Check sheet for the modelled part. Datum: model origin and axes. Units: mm. Coordinates: 2 decimals unless noted, no trailing zeros. Loops run counter-clockwise (first coordinate to the right, second up) from the corner with the lowest first, then second, coordinate; pieces in that order, holes last. Notation, with made-up numbers: M 77,77.25 L 81,77.25 A21 cw 81,105.25 Z; hole C -18.5,81 d6. An arc over 180 degrees is marked long. Use CSV: the item, a comma, the result in double quotes. Start each with the question number.
(1) Go/stop test with flat-tipped pins: pin 1 Ø1.4 at (x, z) = (38.5, 3.5) entering from +Y; pin 2 Ø4 at (x, z) = (37, 3.5) entering from -Y; pin 3 Ø1.5 at (y, z) = (5, 4) entering from -X; pin 4 Ø6 at (x, y) = (-2, -17) entering from +Z. Record where each tip stops, or that it passes through.
(2) Scan lines: line 1 (X direction, y = 3, z = 5.5); line 2 (X direction, y = 2, z = 4.5); line 3 (Z direction, x = 6, y = 3). Record each from-to range of solid material in increasing order.
(3) Section check C-C on y = -17. Record the cut outline in (x, z).
(4) Section check B-B on x = 5. Record the cut outline in (y, z).
(5) Section check A-A on y = 2.5. Record the cut outline in (x, z).
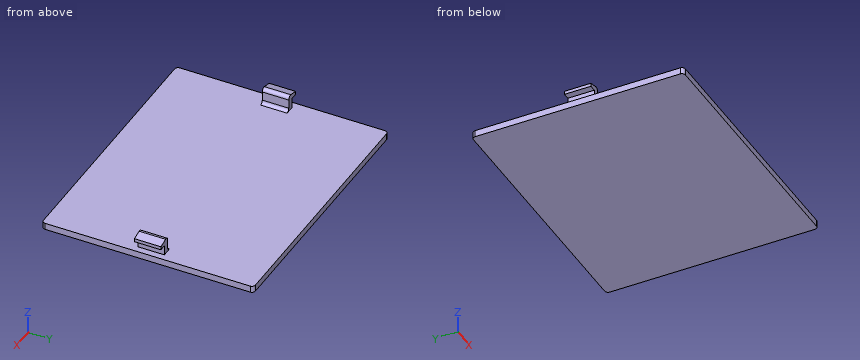
from build123d import *

# Parameters (mm, degrees)
SKETCH_211_W             = 2
SKETCH_211_H             = 8
EXTRUDE_1442_DEPTH       = 2
EXTRUDE_START            = 2
SKETCH_3_W               = 2
SKETCH_3_H               = 8
EXTRUDE_1490_DEPTH       = 3
EXTRUDE_START_2          = 5
SKETCH_4_W               = 2
SKETCH_4_H               = 8
EXTRUDE_1_DEPTH          = 2
CUT_EXTRUDE_2_DEPTH      = 55.219059495
CUT_EXTRUDE_2_DEPTH_BACK = 55.219059495
FILLET_2370_R            = 1
FILLET_4_R               = 1


with BuildPart() as part:
    # Sketch 211 → Extrude 1442 (new body)
    with BuildSketch(Plane.XY):
        Polygon((-38.75749015, -0.345451713), (-38.75749015, -28.345451713), (40.24250985, -28.345451713), (40.24250985, -0.345451713), (38.24250985, -0.345451713), (38.24250985, -26.345451713), (-36.75749015, -26.345451713), (-36.75749015, -0.345451713), align=None)
        with Locations((-37.75749015, 3.654548287)):
            Rectangle(SKETCH_211_W, SKETCH_211_H)
        Polygon((-38.75749015, 35.654548287), (-38.75749015, 7.654548287), (-36.75749015, 7.654548287), (-36.75749015, 33.654548287), (38.24250985, 33.654548287), (38.24250985, 7.654548287), (40.24250985, 7.654548287), (40.24250985, 35.654548287), align=None)
        with Locations((-35.75749015, 3.654548287)):
            Rectangle(SKETCH_211_W, SKETCH_211_H)
        with Locations((37.24250985, 3.654548287)):
            Rectangle(SKETCH_211_W, SKETCH_211_H)
        with Locations((39.24250985, 3.654548287)):
            Rectangle(SKETCH_211_W, SKETCH_211_H)
        Polygon((-34.75749015, -0.345451713), (-36.75749015, -0.345451713), (-36.75749015, -26.345451713), (38.24250985, -26.345451713), (38.24250985, -0.345451713), (36.24250985, -0.345451713), (36.24250985, 7.654548287), (38.24250985, 7.654548287), (38.24250985, 33.654548287), (-36.75749015, 33.654548287), (-36.75749015, 7.654548287), (-34.75749015, 7.654548287), align=None)
    extrude(amount=EXTRUDE_1442_DEPTH)

    # Sketch 3 → Extrude 1490 (add)
    with BuildSketch(Plane.XY.offset(EXTRUDE_START)):
        with Locations((-35.75749015, 3.654548287)):
            Rectangle(SKETCH_3_W, SKETCH_3_H)
        with Locations((37.24250985, 3.654548287)):
            Rectangle(SKETCH_3_W, SKETCH_3_H)
    extrude(amount=EXTRUDE_1490_DEPTH)

    # 基体<4> → 扣子-1 (add)
    with BuildSketch(Plane.XY.offset(EXTRUDE_START_2)):
        with Locations((-37.75749015, 3.654548287)):
            Rectangle(SKETCH_4_W, SKETCH_4_H)
        with Locations((-35.75749015, 3.654548287)):
            Rectangle(SKETCH_4_W, SKETCH_4_H)
        with Locations((37.24250985, 3.654548287)):
            Rectangle(SKETCH_4_W, SKETCH_4_H)
        with Locations((39.24250985, 3.654548287)):
            Rectangle(SKETCH_4_W, SKETCH_4_H)
    extrude(amount=EXTRUDE_1_DEPTH)

    # Sketch 3 2 → 切除-拉伸2 (cut, two sides: drawn at the far end of the back side and taken through both)
    with BuildSketch(Plane(origin=(0, 0, 0), x_dir=(1, 0, 0), z_dir=(0, 1, 0)).offset(-CUT_EXTRUDE_2_DEPTH_BACK)):
        Polygon((-34.75749015, -7), (-38.75749015, -6), (-38.75749015, -7), align=None)
        Polygon((36.24250985, -7), (40.24250985, -6), (40.24250985, -7), align=None)
    extrude(amount=CUT_EXTRUDE_2_DEPTH + CUT_EXTRUDE_2_DEPTH_BACK, mode=Mode.SUBTRACT)

    # Fillet 2370
    fillet_2370_edges = [part.edges().sort_by_distance(p)[0] for p in [
        (40.24250985, -28.345451713, 1),
        (-38.75749015, -28.345451713, 1),
        (-38.75749015, 35.654548287, 1),
        (40.24250985, 35.654548287, 1),
    ]]
    fillet(fillet_2370_edges, radius=FILLET_2370_R)

    # 圆角4
    fillet_4_edges = [part.edges().sort_by_distance(p)[0] for p in [
        (-34.75749015, 3.654548287, 2),
        (36.24250985, 3.654548287, 2),
        (-34.75749015, 3.654548287, 7),
        (36.24250985, 3.654548287, 7),
    ]]
    fillet(fillet_4_edges, radius=FILLET_4_R)


solid = part.part
Outcome:
1,pin 1,"stops at y = 7.65"
1,pin 2,"stops at y = -28.35"
1,pin 3,"stops at x = -36.76"
1,pin 4,"stops at z = 2"
2,line 1,"x = -38.76 to -34.76, 36.24 to 40.24"
2,line 2,"x = -36.76 to -34.76, 36.24 to 38.24"
2,line 3,"z = 0 to 2"
3,outline,"M -38.76,0 L 40.24,0 L 40.24,2 L -38.76,2 Z"
4,outline,"M -28.35,0 L 35.65,0 L 35.65,2 L -28.35,2 Z"
5,outline,"M -38.76,0 L 40.24,0 L 40.24,2 L 38.24,2 L 38.24,5 L 40.24,5 L 40.24,6 L 37.49,6.69 A1 ccw 36.24,5.72 L 36.24,3 A1 cw 35.24,2 L -33.76,2 A1 cw -34.76,3 L -34.76,5.72 A1 ccw -36,6.69 L -38.76,6 L -38.76,5 L -36.76,5 L -36.76,2 L -38.76,2 Z"
